Geometry check sheet. Reference: the model listing, model coordinates, mm. A direction names the side the tool comes from. Round coordinates to 2 decimals unless told otherwise and drop trailing zeros. Loops run counter-clockwise (first coordinate to the right, second up) from the corner with the lowest first, then second, coordinate; pieces in that order, holes last. Notation, with made-up numbers: M 54,-4.5 L 75,-4.5 A25 cw 75,8.5 Z; hole C 43,-3.5 d7. An arc over 180 degrees is marked long. Answer in a Markdown table with one row per item. Add a question column.
```python
from build123d import *

# Parameters (mm, degrees)
F0_W     = 2438.4
F0_H     = 1219.2
F1_DEPTH = 50.8
F3_DEPTH = 1143
F6_DEPTH = 533.4


# Not quite as in the source:
# - a pattern or mirror of a feature is missing from the dataset's text; its kind, count and spacing are read off the source's solid


with BuildPart() as f1:
    # F0 (on Top) → F1 (new body)
    with BuildSketch(Plane.XY):
        Rectangle(F0_W, F0_H)
    extrude(amount=F1_DEPTH)

    # F2 (on Right) → F3 (join, symmetric)
    with BuildSketch(Plane.YZ):
        Polygon((-609.6, -50.8), (-580.2706063252, 0), (-609.6, 0), align=None)
    f3 = extrude(amount=F3_DEPTH, both=True)

    # F3_copies: F3 across plane
    add(f3.mirror(Plane.ZX))

    # F5 (on Front) → F6 (join, symmetric)
    with BuildSketch(Plane.XZ):
        Polygon((1219.2, 0), (1189.8706063252, 0), (1219.2, -50.8), align=None)
    f6 = extrude(amount=F6_DEPTH, both=True)

    # F6_copies: F6 across plane
    add(f6.mirror(Plane(origin=(0, 0, 0), x_dir=(0, 0, -1), z_dir=(-1, 0, 0))))


solid = f1.part
```
1) Go/stop test with flat-tipped pins: pin 1 (14.5 mm diameter, centred on y = -588, z = -23, fed in from -X); pin 2 (10 mm diameter, centred on x = 345.5, y = 301, fed in from -Z); pin 3 (9 mm diameter, centred on y = 601, z = -37, fed in from +X); pin 4 (9 mm diameter, centred on x = 1198, z = -29.5, fed in from +Y). Record where each tip stops, or that it passes through.
2) Draft check along Y on faces 1 (the flat face through (16.002, -595.141, -25.756)), 2 (the flat face through (-17, 609.6, -1)), 3 (the flat face through (-1219.2, -9, -1)), 4 (the flat face through (16.002, 595.141, -25.756)). Enter one of: +Y half, -Y half, draft (parallel to the pull), parting line (faces both ways), or undercut.
3) Thickness scan on L1, parallel to Z at x = 676.5, y = -224.5; L2, parallel to Y at x = -373, z = -13.5; L3, parallel to X at y = -257.5, z = -19. Record the ranges inside material, lowest first. Write a range as [from, to].
4) Cross-section at B-B, the plane z = -34.5. Record the boundary of the cut face in (x, y).
5) Cross-section at C-C, the plane x = 49.5. Record the boundary of the cut face in (y, z), plus the area to 3 significant figures.
6) Set-up check for faces 5 (the flat face through (-17, 9, 50.8)), 6 (the flat face through (-17, 9, 0)), 7 (the flat face through (1204.33, -7.468, -25.044)): record each of +Z, -Z, +X, -X, +Y, -Y from which the full face is reachable in a straight line by a thin tool's end or side.
7) Cross-section at A-A, the plane y = -65.5. Record the boundary of the cut face in (x, z).
Worked answers:
| question | item | result |
|---|---|---|
| 1 | pin 1 | stops at x = -1143 |
| 1 | pin 2 | stops at z = 0 |
| 1 | pin 3 | stops at x = 1143 |
| 1 | pin 4 | passes through |
| 2 | face 1 | undercut |
| 2 | face 2 | +Y half |
| 2 | face 3 | draft |
| 2 | face 4 | undercut |
| 3 | L1 | z = [0, 50.8] |
| 3 | L2 | y = [-609.6, -588.06], [588.06, 609.6] |
| 3 | L3 | x = [-1219.2, -1200.84], [1200.84, 1219.2] |
| 4 | outline | M -1219.2,-533.4 L -1209.79,-533.4 L -1209.79,533.4 L -1219.2,533.4 Z; M -1143,-609.6 L 1143,-609.6 L 1143,-600.19 L -1143,-600.19 Z; M -1143,600.19 L 1143,600.19 L 1143,609.6 L -1143,609.6 Z; M 1209.79,-533.4 L 1219.2,-533.4 L 1219.2,533.4 L 1209.79,533.4 Z |
| 5 | outline | M -609.6,-50.8 L -580.27,0 L 580.27,0 L 609.6,-50.8 L 609.6,50.8 L -609.6,50.8 Z |
| 5 | area | 63,400 mm2 |
| 6 | face 5 | +Z, +X, -X, +Y, -Y |
| 6 | face 6 | -Z |
| 6 | face 7 | -Z, +Y, -Y |
| 7 | outline | M -1219.2,-50.8 L -1189.87,0 L 1189.87,0 L 1219.2,-50.8 L 1219.2,50.8 L -1219.2,50.8 Z |
